Design review of the part built by this model. Coordinates are the model's own, in mm. Face numbers are marked on the shaded views. A direction names the side the tool comes from. Give positions to 0.01 mm unless a question says otherwise; leave off trailing zeros. Loops run counter-clockwise (first coordinate to the right, second up) from the corner with the lowest first, then second, coordinate; pieces in that order, holes last.
from build123d import *

# Parameters (mm, degrees)
BOSS_EXTRUDE3_DEPTH = 25.4
CUT_EXTRUDE2_START  = 2.54
CUT_EXTRUDE2_DEPTH  = 20.32
SKETCH4_W           = 11.045594529
SKETCH4_H           = 88.9
SKETCH4_W_2         = 1.520449279
SKETCH4_H_2         = 82.973089228
BOSS_EXTRUDE4_DEPTH = 11.684
SKETCH6_W           = 1.855490656
SKETCH6_H           = 83.744478267
CUT_EXTRUDE4_DEPTH  = 12.7


with BuildPart() as part:
    # Sketch1 → Boss-Extrude3 (new body)
    with BuildSketch(Plane(origin=(0, 0, 0), x_dir=(0, 0, -1), z_dir=(1, 0, 0))):
        Polygon((-80.07339815, 20.92975129), (-48.153855616, -31.475467797), (-16.234313081, 20.92975129), (9.704221599, 20.92975129), (-22.215320936, -31.475467797), (-0.147855616, -31.475467797), (30.261707149, 18.450680026), (55.407707149, 18.450680026), (66.298249821, 36.330675457), (-29.713750179, 36.330675457), (-48.153855616, 6.055875486), (-66.593961052, 36.330675457), (-89.453961052, 36.330675457), align=None)
    extrude(amount=BOSS_EXTRUDE3_DEPTH)

    # Sketch1<7> → Cut-Extrude2 (cut)
    with BuildSketch(Plane(origin=(0, 0, 0), x_dir=(0, 0, -1), z_dir=(1, 0, 0)).offset(CUT_EXTRUDE2_START)):
        Polygon((-73.682530671, 21.423584358), (-48.153855616, -20.489165733), (-20.954995017, 24.165680026), (17.574318407, 24.165680026), (-12.835244358, -25.760467797), (-3.358557782, -25.760467797), (27.051004983, 24.165680026), (52.197004983, 24.165680026), (56.125638564, 30.615675457), (-26.503048012, 30.615675457), (-48.153855616, -4.930426578), (-69.804663219, 30.615675457), (-79.281349795, 30.615675457), align=None)
    extrude(amount=CUT_EXTRUDE2_DEPTH, mode=Mode.SUBTRACT)

    # Sketch4 → Boss-Extrude4 (add)
    with BuildSketch(Plane(origin=(0, 36.330675457, 0), x_dir=(1, 0, 0), z_dir=(0, 1, 0))):
        with Locations((10.519546417, 14.736249821)):
            Rectangle(SKETCH4_W, SKETCH4_H)
        with Locations((10.202119042, 15.247213808)):
            Rectangle(SKETCH4_W_2, SKETCH4_H_2, mode=Mode.SUBTRACT)
    extrude(amount=-BOSS_EXTRUDE4_DEPTH)

    # Sketch6 → Cut-Extrude4 (cut)
    with BuildSketch(Plane(origin=(0, 36.330675457, 0), x_dir=(1, 0, 0), z_dir=(0, 1, 0))):
        with Locations((10.379765694, 14.977090577)):
            Rectangle(SKETCH6_W, SKETCH6_H)
    extrude(amount=-CUT_EXTRUDE4_DEPTH, mode=Mode.SUBTRACT)


solid = part.part
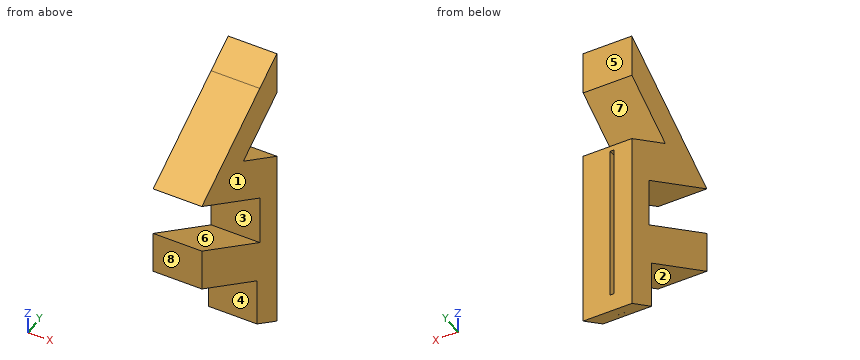
Q1. Draft analysis for pull direction Z (two halves, no side actions). For the marked faces 1, 2 and 3, state which applies: pulls with the +Z half, pulls with the -Z half, needs draft (parallel to the pull), parting line crosses it, or undercut.
Results:
face 1: needs draft
face 2: pulls with the -Z half
face 3: undercut
Q2. Tool access review of the marked faces 4, 5, 6, 7 and 8: name each direction out of +Z, -Z, +X, -X, +Y, -Y from which nothing blocks a thin tool from reaching the whole face with its end or side.
Results:
face 4: -Z, +X, -X, -Y
face 5: +Z, -Z, +X, -X, +Y
face 6: +X, -X
face 7: +X, -X, +Y
face 8: +Z, -Z, +X, -X, -Y
Q3. Take a section at D-D (y = 13). Give the boundary of the cut face in (x, z).
Results:
outline: (0, -26.94) - (25.4, -26.94) - (25.4, -4.87) - (0, -4.87) - close; (0, 21.06) - (25.4, 21.06) - (25.4, 43.92) - (0, 43.92) - close; (0, 52.38) - (25.4, 52.38) - (25.4, 75.24) - (0, 75.24) - close; hole (2.54, -20.25) - (22.86, -20.25) - (22.86, -10.77) - (2.54, -10.77) - close; hole (2.54, 27.76) - (22.86, 27.76) - (22.86, 37.23) - (2.54, 37.23) - close; hole (2.54, 59.08) - (22.86, 59.08) - (22.86, 68.55) - (2.54, 68.55) - close
Q4. Insertion check: pin 1 (2 mm diameter, centred on x = 10, y = 33, fed in from -Z); pin 2 (2 mm diameter, centred on x = 20.5, z = -25.5, fed in from -Y); pin 3 (8 mm diameter, centred on x = 18.5, y = 9.5, fed in from -Z). Each pin has a flat end and moves straight along its axis. Give the tip position at first contact, or say it passes through.
Results:
pin 1: stops at z = -64.88
pin 2: stops at y = 8.99
pin 3: stops at z = -27.25
Q5. Take a section at B-B (x = 7). Give the boundary of the cut face in (y, z) (3 decimals), plus the area to 3 significant figures.
Results:
outline: (-31.475, 0.148) - (18.451, -30.262) - (18.451, -55.408) - (24.647, -59.182) - (24.647, -59.186) - (24.654, -59.186) - (36.331, -66.298) - (36.331, 29.714) - (6.056, 48.154) - (36.331, 66.594) - (36.331, 89.454) - (-31.475, 48.154) - (20.93, 16.234) - (20.93, -9.704) - (-31.475, 22.215) - close; hole (-25.76, 3.359) - (24.166, -27.051) - (24.166, -52.197) - (24.647, -52.49) - (24.647, 29.714) - (25.344, 29.714) - (-4.93, 48.154) - (30.616, 69.805) - (30.616, 79.281) - (-20.489, 48.154) - (24.166, 20.955) - (24.166, -17.574) - (-25.76, 12.835) - close
area: 3,310 mm2
Q6. Wall thickness on line 1 (X direction, y = 32, z = -56.5); line 2 (Y direction, x = 13.25, z = 9.5); line 3 (Z direction, x = 5.5, y = 8.5): over which ranges is each line inside the solid? List them lowest first.
Results:
line 1: x = 0 to 9.45, 11.31 to 25.4
line 2: y = -31.48 to -25.76, -20.28 to -10.6, 20.93 to 24.17, 24.65 to 36.33
line 3: z = -24.2 to -17.51, -8.03 to -2.13, 23.81 to 30.5, 39.97 to 46.67, 49.64 to 56.33, 65.81 to 72.5
Q7. Take a section at A-A (y = -9). Give the boundary of the cut face in (x, z).
Results:
outline: (0, -13.54) - (25.4, -13.54) - (25.4, 8.53) - (0, 8.53) - close; (0, 34.46) - (25.4, 34.46) - (25.4, 61.84) - (0, 61.84) - close; hole (2.54, -6.85) - (22.86, -6.85) - (22.86, 2.63) - (2.54, 2.63) - close; hole (2.54, 41.16) - (22.86, 41.16) - (22.86, 55.15) - (2.54, 55.15) - close
